Read the model definition and answer for the solid it produces. Units are mm, in the model's axes. Coordinates: 2 decimals unless noted, no trailing zeros. Loops run counter-clockwise (first coordinate to the right, second up) from the corner with the lowest first, then second, coordinate; pieces in that order, holes last.
from build123d import *

# Parameters (mm, degrees)
SKETCH1_W           = 250
SKETCH1_H           = 90
BOSS_EXTRUDE1_DEPTH = 15
FILLET1_R           = 10
FILLET2_R           = 5


with BuildPart() as part:
    # Sketch1 → Boss-Extrude1 (new body)
    with BuildSketch(Plane.XY):
        Rectangle(SKETCH1_W, SKETCH1_H)
    extrude(amount=BOSS_EXTRUDE1_DEPTH)

    # Fillet1
    fillet1_edges = [part.edges().sort_by_distance(p)[0] for p in [
        (125, -45, 7.5),
        (-125, -45, 7.5),
        (-125, 45, 7.5),
        (125, 45, 7.5),
    ]]
    fillet(fillet1_edges, radius=FILLET1_R)

    # Fillet2
    fillet2_edges = [part.edges().sort_by_distance(p)[0] for p in [
        (0, 45, 0),
        (0, 45, 15),
        (125, 0, 0),
        (0, -45, 0),
        (-125, 0, 0),
        (-122.071067812, 42.071067812, 0),
        (-122.071067812, -42.071067812, 0),
        (122.071067812, -42.071067812, 0),
        (122.071067812, 42.071067812, 0),
        (125, 0, 15),
        (-125, 0, 15),
        (0, -45, 15),
        (-122.071067812, 42.071067812, 15),
        (-122.071067812, -42.071067812, 15),
        (122.071067812, -42.071067812, 15),
        (122.071067812, 42.071067812, 15),
    ]]
    fillet(fillet2_edges, radius=FILLET2_R)


solid = part.part
Q1. A flat-ended cylindrical pin translates along its axis: pin 1 Ø4 at (y, z) = (29, 2.5) entering from +X. Find the tip coordinate at first contact, or state that the pin passes through.
Findings below:
pin 1: stops at x = 124.97
Q2. Straight lines are drawn through the part: probe 1 along Y at (x, z) = (-64, 4.75); probe 2 along X at (y, z) = (-12, 4.75); probe 3 along X at (y, z) = (-10.5, 11.5). For each, find the intervals that lie inside material, in ascending order.
Findings below:
probe 1: y = -44.99 to 44.99
probe 2: x = -124.99 to 124.99
probe 3: x = -124.77 to 124.77
Q3. A cutting plane is placed at A-A (x = -90). Give the vertices of the cut face in (y, z).
Findings below:
outline: (-45, 5) arc R5 ccw to (-40, 0) - (40, 0) arc R5 ccw to (45, 5) - (45, 10) arc R5 ccw to (40, 15) - (-40, 15) arc R5 ccw to (-45, 10) - close
